Part model, mm, in its own coordinate system. Face numbers are marked on the shaded views. Round coordinates to 2 decimals unless told otherwise and drop trailing zeros. Order: outer loops, then holes, each group sorted by start corner. A loop starts at its lowest first (then second) coordinate and runs counter-clockwise, first axis right, second up. Notation, with made-up numbers: (-3.5, -18) -> (19.5, -18) arc R17 cw to (19.5, 15) -> close; hole circle Ø8 at (-12.75, 62). An arc over 180 degrees is marked (long way). Use CSV: the item, a comma, the result in double quotes.
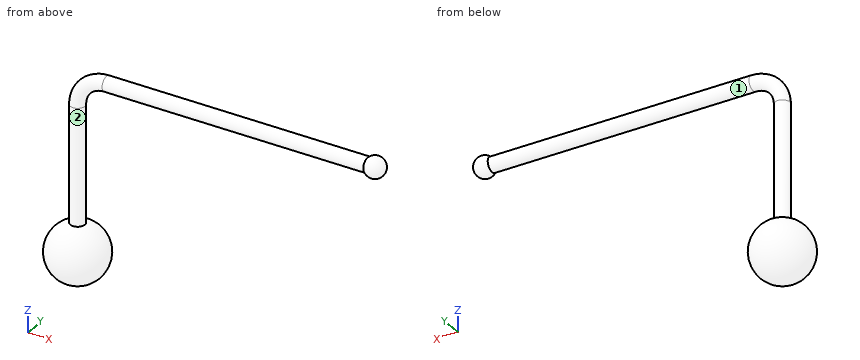
```python
from build123d import *

# Parameters (mm, degrees)
SKETCH2_R         = 2.5
DOME1_FACE_RADIUS = 2.5
DOME1_HEIGHT      = 6


# Read off the part's stored shape, not the designer's step: Dome2
with BuildPart() as part:
    # Sweep1: sweep along a curve in space
    with BuildLine() as sweep1_path:
        Line((0, 0, 0), (0, 0, 40))
        ThreePointArc((10, 0, 50), (2.928932188, 0, 47.071067812), (0, 0, 40))
        Line((10, 0, 50), (100, 0, 50))
    # Sketch2 → Sweep1 (sweep)
    with BuildSketch(Plane.XY):
        Circle(SKETCH2_R)
    sweep(path=sweep1_path.line)

    # Dome1: a dome of height H over a round flat face of radius A is a cap of a sphere of radius (A * A + H * H) / (2 * H)
    dome1_r = (DOME1_FACE_RADIUS * DOME1_FACE_RADIUS + DOME1_HEIGHT * DOME1_HEIGHT) / (2 * DOME1_HEIGHT)
    dome1_base = Plane((100, 0, 50), z_dir=(1, 0, 0))
    with Locations(dome1_base.offset(DOME1_HEIGHT - dome1_r)):
        dome1_ball = Sphere(dome1_r, mode=Mode.PRIVATE)
    add(split(dome1_ball, bisect_by=dome1_base, keep=Keep.TOP, mode=Mode.PRIVATE))

    # Dome2 outline → Dome2 (revolve)
    with BuildSketch(Plane.XZ):
        with BuildLine():
            Line((0, 3e-09), (0, -20))
            ThreePointArc((0, -20), (10.077822186, -11.10347777), (2.499999995, 2e-09))
            Line((2.499999995, 2e-09), (0, 3e-09))
        make_face()
    revolve(axis=Axis((0, 0, 0), (0, 0, 1)))


solid = part.part
```
(1) Cut at A-A, the plane z = 17.5. Give the cut face in (x, y).
Reply:
outline,"circle Ø5 at (0, 0)"
(2) Pull direction X, two halves, no side cores. Call the marked faces 1 and 2: released by +X, released by -X, zero draft, split by the parting line, or undercut.
Reply:
face 1,"undercut"
face 2,"split by the parting line"
(3) Probe probe 1 along Z at (x, y) = (9, -0.75); probe 2 along Z at (x, y) = (41, 0.25); probe 3 along X at (y, z) = (-1, -4). List the from-to ranges inside material, lowest first. Write a range as [from, to].
Reply:
probe 1,"[-14.49, -5.2], [47.55, 52.34]"
probe 2,"[47.51, 52.49]"
probe 3,"[-8.25, 8.25]"
(4) Cut at B-B, the plane x = 20. Give the cut face in (y, z).
Reply:
outline,"circle Ø5 at (0, 50)"
(5) Drop flat-ended pins along their axis: P1, Ø8, axis at y = -1.5, z = 6.5, coming from the -X side; P2, Ø12, axis at x = 19, z = 43.5, coming from the -Y side; P3, Ø8, axis at x = 8, y = -1.5, coming from the -Z side. Give the stop position or say it passes through.
Reply:
P1,"x = -2.5"
P2,"y = -2.45"
P3,"z = -19.12"
